Geometry check sheet. Reference: drawing and pictorial views, mm from the part's lowest x, y, z. Give positions to 0.01 mm unless a question says otherwise; leave off trailing zeros. Write each loop counter-clockwise with the first axis right and the second up, starting at its lowest first coordinate (ties: lowest second). Pieces come first, ordered by that corner, then holes. Notation, with made-up numbers: (-3, 62.25) -> (43, 62.25) arc R17 ccw to (43, 83.25) -> close; hole circle Ø11 at (39, 1). An arc over 180 degrees is marked (long way). Use a Markdown table: item, result. Add a question column.
1. Scan lines: probe 1 along Y at (x, z) = (23, 0.55); probe 2 along X at (y, z) = (50, 0.1) (1 decimal); probe 3 along Y at (x, z) = (61.5, 1.3) (1 decimal). Record each from-to range of solid material in increasing order. Write a range as [from, to].
2. Gauge pin test, flat ends, axial feed: P1, Ø0.8, axis at y = 48.5, z = 0.5, coming from the +X side; P2, Ø0.8, axis at y = 46.5, z = 0.5, coming from the -X side. Record the tip position at first contact, or that the pin passes through.
3. Cross-section at A-A (z = 0.95). Count the separate pieces of the cut face and the enclosed holes in it, then the cut area to 3 significant figures.
4. Cross-section at B-B (y = 45.5). Enter the section's corners in (x, z) (1 decimal), then the cut area to 3 significant figures.
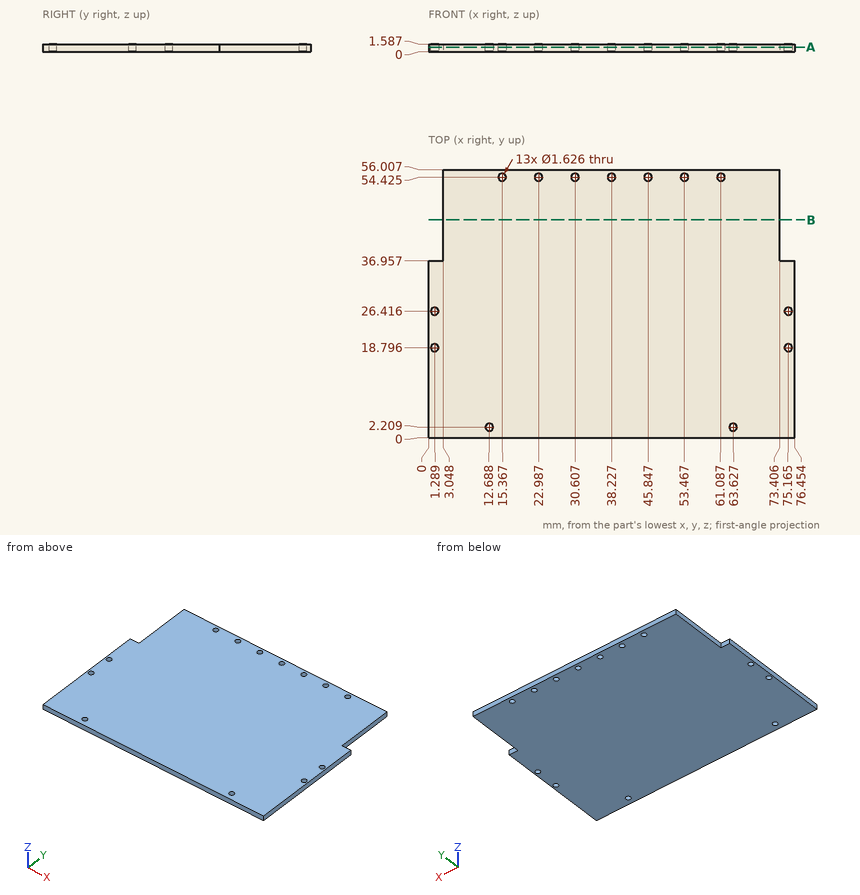
Worked answers:
| question | item | result |
|---|---|---|
| 1 | probe 1 | y = [0, 53.61], [55.24, 56.01] |
| 1 | probe 2 | x = [3, 73.4] |
| 1 | probe 3 | y = [0, 53.7], [55.1, 56] |
| 2 | P1 | stops at x = 73.41 |
| 2 | P2 | stops at x = 3.05 |
| 3 | separate pieces | 1 |
| 3 | enclosed holes | 13 |
| 3 | area | 4,140 mm² |
| 4 | outline | (3, 0) -> (73.4, 0) -> (73.4, 1.6) -> (3, 1.6) -> close |
| 4 | area | 112 mm² |
